Input: part model. Units: mm. Frame: model coordinates. A direction names the side the tool comes from. Round coordinates to 2 decimals unless told otherwise and drop trailing zeros. Write each loop counter-clockwise with the first axis right and the second up, starting at its lowest first coordinate (ties: lowest second). Pieces come first, ordered by that corner, then holes. Notation, with made-up numbers: (25.25, 23.5) -> (45.25, 23.5) arc R16 ccw to (45.25, 41.5) -> close; hole circle Ø6 at (70, 42). An arc over 180 degrees is marked (long way). Write item = value, one per line.
```python
from build123d import *

# Parameters (mm, degrees)
SKETCH_W        = 100
SKETCH_H        = 64
SKETCH_R        = 3.2
SKETCH_R_2      = 1.8
SKETCH_R_3      = 4
PAD_DEPTH       = 15
SKETCH001_R     = 11.2
SKETCH001_R_2   = 6
POCKET_DEPTH    = 5.4
SKETCH002_R     = 3.2
POCKET001_DEPTH = 3.2


with BuildPart() as part:
    # Sketch → Pad (new body)
    with BuildSketch(Plane.XY):
        with Locations((50, 32)):
            Rectangle(SKETCH_W, SKETCH_H)
        with Locations((50, 42.85)):
            Circle(SKETCH_R, mode=Mode.SUBTRACT)
        with Locations((65.5, 58.35)):
            Circle(SKETCH_R_2, mode=Mode.SUBTRACT)
        with Locations((65.5, 27.35)):
            Circle(SKETCH_R_2, mode=Mode.SUBTRACT)
        with Locations((34.5, 27.35)):
            Circle(SKETCH_R_2, mode=Mode.SUBTRACT)
        with Locations((34.5, 58.35)):
            Circle(SKETCH_R_2, mode=Mode.SUBTRACT)
        with Locations((20, 10)):
            Circle(SKETCH_R, mode=Mode.SUBTRACT)
        with Locations((80, 10)):
            Circle(SKETCH_R, mode=Mode.SUBTRACT)
        with Locations((82, 42.85)):
            Circle(SKETCH_R_3, mode=Mode.SUBTRACT)
        with Locations((18, 42.85)):
            Circle(SKETCH_R_3, mode=Mode.SUBTRACT)
    extrude(amount=PAD_DEPTH)

    # Sketch001 (on Face15 of Pad) → Pocket (cut)
    with BuildSketch(Plane.XY.offset(15)):
        with Locations((50, 42.85)):
            Circle(SKETCH001_R)
        with Locations((20, 10)):
            Circle(SKETCH001_R_2)
        with Locations((80, 10)):
            Circle(SKETCH001_R_2)
    extrude(amount=-POCKET_DEPTH, mode=Mode.SUBTRACT)

    # Sketch002 (on Face4 of Pocket) → Pocket001 (cut)
    with BuildSketch(Plane(origin=(0, 0, 0), x_dir=(1, 0, 0), z_dir=(0, 0, -1))):
        with Locations((34.5, -27.35)):
            Circle(SKETCH002_R)
        with Locations((65.5, -27.35)):
            Circle(SKETCH002_R)
        with Locations((34.5, -58.35)):
            Circle(SKETCH002_R)
        with Locations((65.5, -58.35)):
            Circle(SKETCH002_R)
    extrude(amount=-POCKET001_DEPTH, mode=Mode.SUBTRACT)


solid = part.part
```
1) Cut plane D-D (y = 27.35). Return the cut outline in (x, z), and give its area (3 significant figures).
Solutions:
outline = (0, 0) -> (31.3, 0) -> (31.3, 3.2) -> (32.7, 3.2) -> (32.7, 15) -> (0, 15) -> close; (36.3, 3.2) -> (37.7, 3.2) -> (37.7, 0) -> (62.3, 0) -> (62.3, 3.2) -> (63.7, 3.2) -> (63.7, 15) -> (36.3, 15) -> close; (67.3, 3.2) -> (68.7, 3.2) -> (68.7, 0) -> (100, 0) -> (100, 15) -> (67.3, 15) -> close
area = 1,370 mm^2
2) Line query: L1, parallel to X at y = 27.35, z = 1.75; L2, parallel to Y at x = 34.5, z = 9.75; L3, parallel to Y at x = 21, z = 4.75. Output: solid intervals per line, ascending. Write a range as from..to.
Solutions:
L1 = 0..31.3, 37.7..62.3, 68.7..100
L2 = 0..25.55, 29.15..56.55, 60.15..64
L3 = 0..6.96, 13.04..40.2, 45.5..64
3) Draft query along Y for faces 1 (the face through (49, 64, 7)), 2 (the face through (22.769, 4.677, 12.338)), 3 (the face through (49, 0, 7)). Return one class per face: +Y half, -Y half, draft (parallel to the pull), parting line (faces both ways), or undercut.
Solutions:
face_1 = +Y half
face_2 = undercut
face_3 = -Y half
4) Cut plane B-B (x = 50). Return the cut outline in (y, z).
Solutions:
outline = (0, 0) -> (39.65, 0) -> (39.65, 9.6) -> (31.65, 9.6) -> (31.65, 15) -> (0, 15) -> close; (46.05, 0) -> (64, 0) -> (64, 15) -> (54.05, 15) -> (54.05, 9.6) -> (46.05, 9.6) -> close
5) Access query for faces 4 (the face through (67, 60, 3.2)), 5 (the face through (83, 7, 9.6)), 6 (the face through (16.8, 10.1, 4.7)). Directions: +Z, -Z, +X, -X, +Y, -Y. A direction counts if a zero-diameter tool reaches every point of the face in a straight line with its end or side. Return the directions, or none.
Solutions:
face_4 = -Z
face_5 = +Z
face_6 = +Z, -Z
6) Cut plane C-C (z = 12.5). Count the separate pieces of the cut face and the enclosed holes in it, and give its area (3 significant figures).
Solutions:
separate_pieces = 1
enclosed_holes = 9
area = 5,640 mm^2
7) First-contact query: P1, Ø5, axis at x = 80, y = 10, coming from the -Z side; P2, Ø6, axis at x = 65.5, y = 27.35, coming from the -Z side. Flat tips, straight axial feed; report the tip coordinate or a pass-through.
Solutions:
P1 = through
P2 = 3.2
8) Cut plane A-A (y = 42.85). Return the cut outline in (x, z).
Solutions:
outline = (0, 0) -> (14, 0) -> (14, 15) -> (0, 15) -> close; (22, 0) -> (46.8, 0) -> (46.8, 9.6) -> (38.8, 9.6) -> (38.8, 15) -> (22, 15) -> close; (53.2, 0) -> (78, 0) -> (78, 15) -> (61.2, 15) -> (61.2, 9.6) -> (53.2, 9.6) -> close; (86, 0) -> (100, 0) -> (100, 15) -> (86, 15) -> close
